Input: dimensioned drawing with shaded views. Units: mm. Origin: part minimum x, y, z. A direction names the side the tool comes from. Round coordinates to 2 decimals unless told otherwise and drop trailing zeros. Loops run counter-clockwise (first coordinate to the right, second up) from the corner with the lowest first, then second, coordinate; pieces in that order, holes last. Notation, with made-up numbers: (66.25, -30.75) - (96.25, -30.75) arc R15 ccw to (96.25, -4.75) - close; hole circle Ø11 at (23.25, 80). An arc over 180 degrees is marked (long way). One line per question, with ' | ' between items. Start each with the question number.
Item 1: Section B-B, the plane y = 49. Return loops of the section in (x, z), plus the area to 3 significant figures.
Item 2: First-contact query: pin 1 (1 mm diameter, centred on x = 1, y = 31, fed in from +Z). Flat tip, straight axial feed; report the tip coordinate or a pass-through.
Item 3: Material intervals for line 1 along Y through (x, z) = (29, 20.75); line 2 along X through (y, z) = (39, 8.5); line 3 along Z through (x, y) = (47, 17.5), sorted ascending.
Item 4: Draft query along Y for the marked faces 3, 4 and 5. Return one class per face: pulls with the +Y half, pulls with the -Y half, needs draft (parallel to the pull), parting line crosses it, or undercut.
Item 5: Section A-A, the plane z = 4. Return loops of the section in (x, y).
Item 6: Set-up query: the marked faces 1 and 2. Return all of +Z, -Z, +X, -X, +Y, -Y with unobstructed straight access to the full face (end or side cutting, diameter ignored); none if empty.
Item 7: Section C-C, the plane x = 68. Return loops of the section in (y, z).
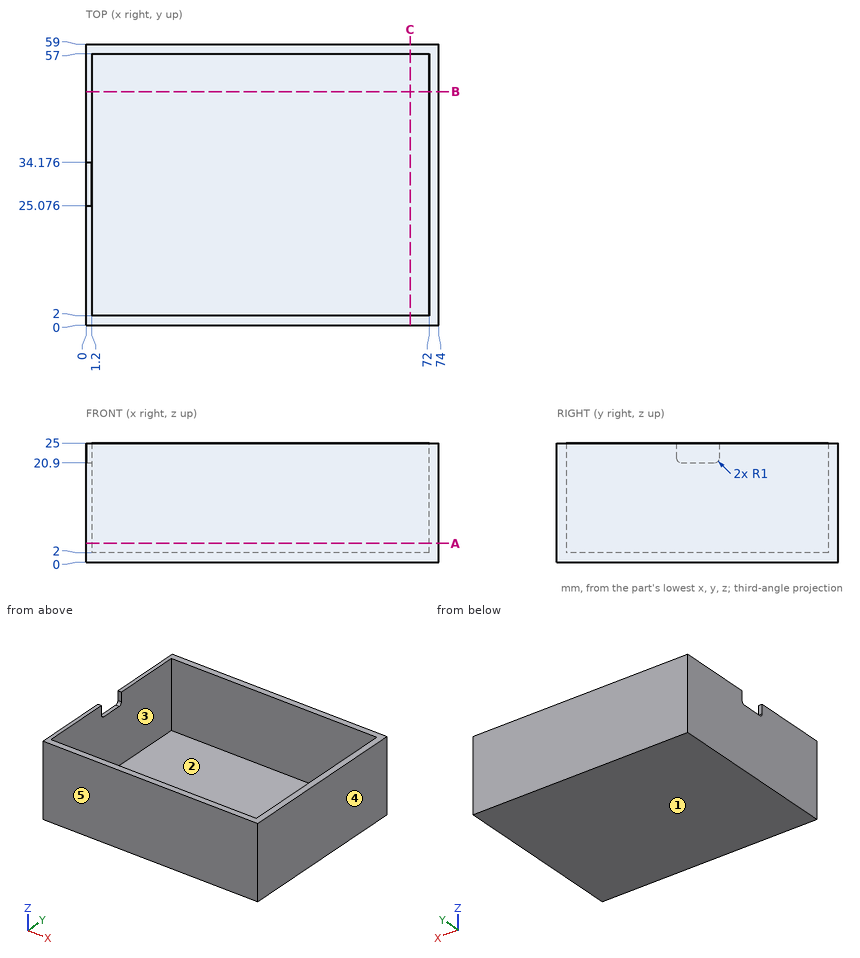
Return value:
1) outline: (0, 0) - (74, 0) - (74, 25) - (72, 25) - (72, 2) - (1.2, 2) - (1.2, 25) - (0, 25) - close | area: 222 mm2
2) pin 1: z = 20.9
3) line 1: 0 to 2, 57 to 59 | line 2: 0 to 1.2, 72 to 74 | line 3: 0 to 2
4) face 3: undercut | face 4: needs draft | face 5: pulls with the -Y half
5) outline: (0, 0) - (74, 0) - (74, 59) - (0, 59) - close; hole (1.2, 2) - (72, 2) - (72, 57) - (1.2, 57) - close
6) face 1: -Z, +X, -X, +Y, -Y | face 2: +Z
7) outline: (0, 0) - (59, 0) - (59, 25) - (57, 25) - (57, 2) - (2, 2) - (2, 25) - (0, 25) - close
